from build123d import *

# Parameters (mm, degrees)
BOSS_EXTRUDE1_DEPTH = 0.8
SKETCH3_W           = 10
SKETCH3_H           = 0.8
CUT_EXTRUDE1_DEPTH  = 1.8


with BuildPart() as part:
    # Sketch2 → Boss-Extrude1 (new body)
    with BuildSketch(Plane(origin=(0, 0, 0), x_dir=(1, 0, 0), z_dir=(0, 1, 0))):
        Polygon((0, 69.507859614), (-60.195572189, 34.753929807), (-60.195572189, -34.753929807), (0, -69.507859614), (60.195572189, -34.753929807), (60.195572189, 34.753929807), align=None)
    extrude(amount=BOSS_EXTRUDE1_DEPTH)

    # Sketch3 → Cut-Extrude1 (cut, through all)
    with BuildSketch(Plane.XZ):
        Polygon((29.664773392, -52.380894711), (24.664773392, -43.720640673), (25.357593716, -43.320640673), (30.357593716, -51.980894711), align=None)
        with Locations((55.195572189, -0.1)):
            Rectangle(SKETCH3_W, SKETCH3_H)
        Polygon((-30.530798796, -51.880894711), (-25.530798796, -43.220640673), (-24.837978473, -43.620640673), (-29.837978473, -52.280894711), align=None)
        with Locations((-55.195572189, 0.1)):
            Rectangle(SKETCH3_W, SKETCH3_H)
        Polygon((-29.664773392, 52.380894711), (-24.664773392, 43.720640673), (-25.357593716, 43.320640673), (-30.357593716, 51.980894711), align=None)
        Polygon((30.530798796, 51.880894711), (25.530798796, 43.220640673), (24.837978473, 43.620640673), (29.837978473, 52.280894711), align=None)
    extrude(amount=-CUT_EXTRUDE1_DEPTH, mode=Mode.SUBTRACT)


solid = part.part
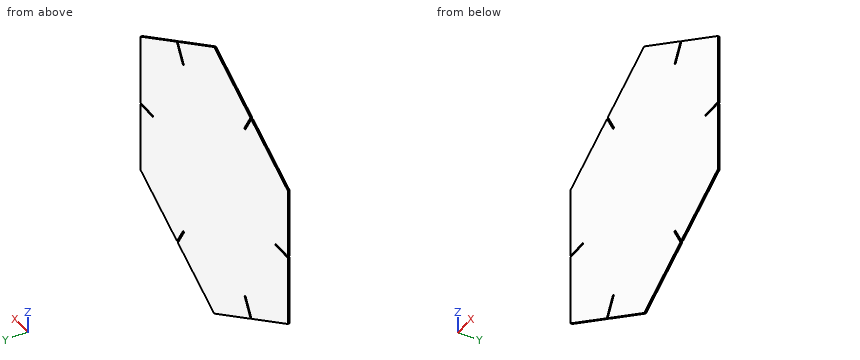
The listing builds one solid part. Answer for the finished solid, in the listing's coordinates (mm). Give positions to 0.01 mm unless a question says otherwise; leave off trailing zeros. Write each loop counter-clockwise with the first axis right and the second up, starting at its lowest first coordinate (ties: lowest second). Pieces come first, ordered by that corner, then holes.
Item 1: Find the intervals of material crossed by line 1 along X through (y, z) = (0.7, 0); line 2 along Z through (x, y) = (29, 0.4); line 3 along Z through (x, y) = (-53.5, 0.5), in increasing order.
Item 2: Section B-B, the plane x = 39 is taken. Write down the section's boundary in (y, z), plus the area to 3 significant figures.
Item 3: Section C-C, the plane z = 41 is taken. Write down the section's boundary in (x, y), plus the area to 3 significant figures.
Completed:
1. line 1: x = -50.2 to 50.2
1. line 2: z = -52.76 to -51.23, -49.63 to 49.23, 50.83 to 52.76
1. line 3: z = -38.62 to -0.3, 0.5 to 38.62
2. outline: (0, -46.99) - (0.8, -46.99) - (0.8, 46.99) - (0, 46.99) - close
2. area: 75.2 mm2
3. outline: (-49.38, 0) - (49.38, 0) - (49.38, 0.8) - (-49.38, 0.8) - close
3. area: 79.0 mm2
